The listing builds one solid part. Answer for the finished solid, in the listing's coordinates (mm). Round coordinates to 2 decimals unless told otherwise and drop trailing zeros. Write each loop counter-clockwise with the first axis right and the second up, starting at its lowest first coordinate (ties: lowest second). Pieces come first, ordered by that corner, then holes. Notation, with made-up numbers: M 24.25,54 L 42.25,54 A17 cw 42.25,63 Z; hole C 48,-9.5 d11. An arc over 180 degrees is marked long. One line per item, written item: value. Start each with the question number.
(1) Section B-B (x = 9.5) is taken. Determine the outline of the cut face in (y, z).
(2) Consider probe 1 along Z at (x, y) = (0, 0.8); probe 2 along Z at (x, y) = (9, 1.25); probe 3 along Z at (x, y) = (-11, 0.5). Determine where each line is inside the solid, lowest interval first.
(3) For a pull along Z with two mould halves and no side action, classify faces 1 (the cylindrical face through (-8.2, 0.8, 0.6)), 2 (the cylindrical face through (-12.22, 0.8, -12.25)), 3 (the flat face through (-12.7, 1, 0)) as released by +Z, released by -Z, zero draft, split by the parting line, or undercut.
(4) Section D-D (y = 0.9) is taken. State how many separate pieces and enclosed holes the cut face has, plus the area to 3 significant figures.
(5) Section C-C (z = 3) is taken. Determine the outline of the cut face in (x, y).
(6) Section A-A (z = 0) is taken. Determine the outline of the cut face in (x, y).
Autodesk Inventor part; units mm, degrees
ref_plane "YZ Plane" through (0, 0, 0) normal (1, 0, 0) x (0, 1, 0)
ref_plane "XZ Plane" through (0, 0, 0) normal (0, 1, 0) x (-1, 0, 0)
ref_plane "XY Plane" through (0, 0, 0) normal (0, 0, 1) x (1, 0, 0)
sketch "Sketch1" plane through (0, 0, 0) normal (0, 1, 0) x (-1, 0, 0)
  line L0 (-12.7, 12.7) -> (12.7, 12.7)
  line L1 (12.7, 12.7) -> (12.7, -12.7)
  line L2 (12.7, -12.7) -> (-12.7, -12.7)
  line L3 (-12.7, -12.7) -> (-12.7, 12.7)
  line L4 (-12.7, 12.7) -> (12.7, -12.7) construction
  line L5 (12.7, 12.7) -> (-12.7, -12.7) construction
  line L6 (-9.525, 9.525) -> (9.525, 9.525) construction
  line L7 (9.525, 9.525) -> (9.525, -9.525) construction
  line L8 (9.525, -9.525) -> (-9.525, -9.525) construction
  line L9 (-9.525, -9.525) -> (-9.525, 9.525) construction
  line L10 (-9.525, 9.525) -> (9.525, -9.525) construction
  line L11 (9.525, 9.525) -> (-9.525, -9.525) construction
  circle A0 centre (9.525, 9.525) radius 1.7526
  circle A1 centre (-9.525, 9.525) radius 1.7526
  circle A2 centre (-9.525, -9.525) radius 1.7526
  circle A3 centre (9.525, -9.525) radius 1.7526
  circle A4 centre (0, 0) radius 7
  circle A5 centre (0, 0) radius 9 construction
  line L12 (9, 0) -> (0, 0) construction
  circle A6 centre (9, 0) radius 1
  circle A7 centre (0, 9) radius 1
  circle A8 centre (-9, 0) radius 1
  circle A9 centre (0, -9) radius 1
  dimension "d10" = 18
  dimension "d0" = 25.4
  dimension "d1" = 25.4
  dimension "d2" = 19.05
  dimension "d3" = 19.05
  dimension "d4" = 3.5052
  dimension "d7" = 360
  dimension "d9" = 14
  dimension "d11" = 2
  dimension "d14" = 360
extrude "Extrusion1" add sketch "Sketch1" along normal blind 1.5875
fillet "Fillet1" radius 1.5875 4 edges at (-12.7, 0.7937, 12.7) (12.7, 0.7937, 12.7) (-12.7, 0.7937, -12.7) (12.7, 0.7937, -12.7)
properties part number "Drive Plate"
Recorded:
1. outline: M 0,-12.7 L 1.59,-12.7 L 1.59,-11.28 L 0,-11.28 Z; M 0,-7.77 L 1.59,-7.77 L 1.59,-0.87 L 0,-0.87 Z; M 0,0.87 L 1.59,0.87 L 1.59,7.77 L 0,7.77 Z; M 0,11.28 L 1.59,11.28 L 1.59,12.7 L 0,12.7 Z
2. probe 1: z = -12.7 to -10, -8 to -7, 7 to 8, 10 to 12.7
2. probe 2: z = -12.7 to -11.2, -7.85 to -1, 1 to 7.85, 11.2 to 12.7
2. probe 3: z = -12.7 to -10.47, -8.58 to 8.58, 10.47 to 12.7
3. face 1: undercut
3. face 2: released by -Z
3. face 3: zero draft
4. separate pieces: 1
4. enclosed holes: 9
4. area: 438 mm2
5. outline: M -12.7,0 L -6.32,0 L -6.32,1.59 L -12.7,1.59 Z; M 6.32,0 L 12.7,0 L 12.7,1.59 L 6.32,1.59 Z
6. outline: M -12.7,0 L -10,0 L -10,1.59 L -12.7,1.59 Z; M -8,0 L -7,0 L -7,1.59 L -8,1.59 Z; M 7,0 L 8,0 L 8,1.59 L 7,1.59 Z; M 10,0 L 12.7,0 L 12.7,1.59 L 10,1.59 Z
